from build123d import *

# Parameters (mm, degrees)
BOSS_EXTRUDE1_DEPTH = 30
SKETCH6_W           = 15
SKETCH6_H           = 30
BOSS_EXTRUDE2_DEPTH = 24


with BuildPart() as part:
    # Sketch2 → Boss-Extrude1 (new body)
    with BuildSketch(Plane.XY):
        Polygon((-35.659220441, 48.994166095), (20.212047263, 48.994166095), (3.020324726, 8.994166095), (36.417587641, -13.019984577), (36.417587641, -68.485610583), (19.225865104, -108.485610583), (33.318130441, -145.920995684), (-101.80917988, -146.898605829), (-88.260031439, -109.263242453), (-106.02870282, -69.516171603), (-106.831218915, -14.056351587), (-73.755968311, 8.438710038), (-91.524639692, 48.185780888), align=None)
    extrude(amount=BOSS_EXTRUDE1_DEPTH)

    # Sketch6 → Boss-Extrude2 (add)
    with BuildSketch(Plane(origin=(0, 0, 0), x_dir=(0, 0, -1), z_dir=(1, 0, 0))):
        with Locations((-14.441506787, -108.571370402)):
            Rectangle(SKETCH6_W, SKETCH6_H)
    extrude(amount=BOSS_EXTRUDE2_DEPTH)


solid = part.part
Check sheet for the modelled part. Datum: model origin and axes. Units: mm. A direction names the side the tool comes from. Coordinates: 2 decimals unless noted, no trailing zeros. Write each loop counter-clockwise with the first axis right and the second up, starting at its lowest first coordinate (ties: lowest second). Pieces come first, ordered by that corner, then holes. Notation, with made-up numbers: M 66.5,25.5 L 78.5,25.5 A14 cw 78.5,40.5 Z; hole C 83.5,1 d6. An arc over 180 degrees is marked long. Answer as CSV lines item,"result".
Q1. Cross-section at B-B (z = 11). Record the boundary of the cut face in (x, y), then the cut area to 3 significant figures.
Check result:
outline,"M -106.83,-14.06 L -106.03,-69.52 L -88.26,-109.26 L -101.81,-146.9 L 33.32,-145.92 L 24,-121.17 L 24,-97.38 L 36.42,-68.49 L 36.42,-13.02 L 3.02,8.99 L 20.21,48.99 L -35.66,48.99 L -91.52,48.19 L -73.76,8.44 Z"
area,"23,700 mm^2"
Q2. Cross-section at C-C (y = -115). Record the boundary of the cut face in (x, z), then the cut area to 3 significant figures.
Check result:
outline,"M -90.33,0 L 21.68,0 L 21.68,6.94 L 24,6.94 L 24,21.94 L 21.68,21.94 L 21.68,30 L -90.33,30 Z"
area,"3,390 mm^2"
Q3. Mould release check, pull along Y, two halves, no side actions. Record for faces 5 (the face through (-34, -48, 30)), 6 (the face through (23, -109, 21.942)), 7 (the face through (-8, 48.994, 15)): released by +Y, released by -Y, zero draft, split by the parting line, or undercut.
Check result:
face 5,"zero draft"
face 6,"undercut"
face 7,"released by +Y"
Q4. Material ranges on probe 1 along Y at (x, z) = (10, 16); probe 2 along Y at (x, z) = (10.5, 20.5); probe 3 along X at (y, z) = (-23, 2.5), recorded low to high. Write a range as from..to.
Check result:
probe 1,"-146.09..4.39, 25.23..48.99"
probe 2,"-146.09..4.06, 26.4..48.99"
probe 3,"-106.7..36.42"
Q5. Go/stop test with flat-tipped pins: pin 1 (10 mm diameter, centred on y = 11.5, z = 20, fed in from +X); pin 2 (12 mm diameter, centred on y = -48.5, z = 12, fed in from -X); pin 3 (4 mm diameter, centred on x = 22, y = -109.5, fed in from -Z). Record where each tip stops, or that it passes through.
Check result:
pin 1,"x = 6.8"
pin 2,"x = -106.42"
pin 3,"z = 6.94"
Q6. Set-up check for faces 1 (the face through (-90.53, -2.97, 14.79)), 2 (the face through (-34, -48, 0)), 3 (the face through (19.49, -1.86, 14.79)), 4 (the face through (23, -109, 6.942)): record each of +Z, -Z, +X, -X, +Y, -Y from which the full face is reachable in a straight line by a thin tool's end or side.
Check result:
face 1,"+Z, -Z, -X"
face 2,"-Z, +X, -X, +Y, -Y"
face 3,"+Z, -Z, +X"
face 4,"-Z, +X"
Q7. Cross-section at D-D (y = 15). Record the boundary of the cut face in (x, z).
Check result:
outline,"M -76.69,0 L 5.6,0 L 5.6,30 L -76.69,30 Z"
Q8. Cross-section at A-A (x = -85). Record the boundary of the cut face in (y, z), then the cut area to 3 significant figures.
Check result:
outline,"M -146.78,0 L 0.79,0 L 0.79,30 L -146.78,30 Z; M 33.59,0 L 48.28,0 L 48.28,30 L 33.59,30 Z"
area,"4,870 mm^2"
